Read the model definition and answer for the solid it produces. Units are mm, in the model's axes. A direction names the side the tool comes from. Coordinates: 2 decimals unless noted, no trailing zeros. Order: outer loops, then holes, each group sorted by start corner. A loop starts at its lowest first (then second) coordinate and runs counter-clockwise, first axis right, second up. Notation, with made-up numbers: (32, 70.5) -> (52, 70.5) arc R12 ccw to (52, 78.5) -> close; hole circle Ø5 at (-5, 69.25). An arc over 180 degrees is marked (long way). Use CSV: the item, a comma, the result in double quotes.
```python
from build123d import *

# Parameters (mm, degrees)
SKETCH_1_W           = 180
SKETCH_1_H           = 60
SKETCH_1_R           = 11
SKETCH_1_R_2         = 1.5
EXTRUDE_3_DEPTH      = 5
SKETCH_2_W           = 10
SKETCH_2_H           = 20
EXTRUDE_4_DEPTH      = 20
SKETCH_4_R           = 4
CUT_EXTRUDE_1_DEPTH  = 20
SKETCH_8_W           = 3
SKETCH_8_H           = 20
CUT_EXTRUDE_4_DEPTH  = 10
SKETCH_10_W          = 14
SKETCH_10_H          = 20
EXTRUDE_5_DEPTH      = 10
SKETCH_9_R           = 4
CUT_EXTRUDE_5_DEPTH  = 10
SKETCH_12_W          = 13.5
SKETCH_12_H          = 20
CUT_EXTRUDE_6_DEPTH  = 10
SKETCH_15_W          = 1
SKETCH_15_H          = 20
CUT_EXTRUDE_7_DEPTH  = 10
FILLET_5_R           = 5
SKETCH_21_W          = 10
SKETCH_21_H          = 18
EXTRUDE_6_DEPTH      = 20
SKETCH_23_R          = 4
CUT_EXTRUDE_9_DEPTH  = 20
FILLET_8_R           = 8
SKETCH_25_W          = 11.311173877
SKETCH_25_H          = 1.5
CUT_EXTRUDE_10_DEPTH = 20
FILLET_9_R           = 8
SKETCH_28_W          = 10
SKETCH_28_H          = 16.5
EXTRUDE_7_DEPTH      = 25
SKETCH_31_W          = 27.629977972
SKETCH_31_H          = 33.342762348
CUT_EXTRUDE_12_DEPTH = 20
SKETCH_33_W          = 10
SKETCH_33_H          = 20
EXTRUDE_8_DEPTH      = 6
SKETCH_34_W          = 10
SKETCH_34_H          = 20
CUT_EXTRUDE_13_DEPTH = 6
SKETCH_35_R          = 4
CUT_EXTRUDE_14_DEPTH = 10
FILLET_11_R          = 8
SKETCH_36_R          = 1.5
CUT_EXTRUDE_15_DEPTH = 10
SKETCH_37_R          = 4.5
CUT_EXTRUDE_16_DEPTH = 10
SKETCH_38_R          = 11.5
CUT_EXTRUDE_17_DEPTH = 10
SKETCH_39_R          = 1.5
CUT_EXTRUDE_18_DEPTH = 10
FILLET_13_R          = 8


with BuildPart() as part:
    # 스케치1 → 보스-돌출3 (new body)
    with BuildSketch(Plane(origin=(0, 0, 0), x_dir=(1, 0, 0), z_dir=(0, 1, 0))):
        with Locations((36.632340007, -1.742375967)):
            Rectangle(SKETCH_1_W, SKETCH_1_H)
        with Locations(Location((105.632340007, 7.257624033, 0), (0, 0, 270))):
            Circle(SKETCH_1_R, mode=Mode.SUBTRACT)
        with Locations(Location((90.132340007, 22.757624033, 0), (0, 0, 270))):
            Circle(SKETCH_1_R_2, mode=Mode.SUBTRACT)
        with Locations(Location((121.132340007, 22.757624033, 0), (0, 0, 270))):
            Circle(SKETCH_1_R_2, mode=Mode.SUBTRACT)
        with Locations(Location((90.132340007, -8.242375967, 0), (0, 0, 270))):
            Circle(SKETCH_1_R_2, mode=Mode.SUBTRACT)
        with Locations(Location((121.132340007, -8.242375967, 0), (0, 0, 270))):
            Circle(SKETCH_1_R_2, mode=Mode.SUBTRACT)
        with Locations(Location((-32.617755763, 4.712595626, 0), (0, 0, 270))):
            Circle(SKETCH_1_R_2, mode=Mode.SUBTRACT)
        with Locations(Location((-45.654401225, 19.548720133, 0), (0, 0, 270))):
            Circle(SKETCH_1_R_2, mode=Mode.SUBTRACT)
        with Locations(Location((-45.654401225, -10.123528882, 0), (0, 0, 270))):
            Circle(SKETCH_1_R_2, mode=Mode.SUBTRACT)
    extrude(amount=EXTRUDE_3_DEPTH)

    # 스케치2 → 보스-돌출4 (add)
    with BuildSketch(Plane(origin=(0, 5, 0), x_dir=(1, 0, 0), z_dir=(0, 1, 0))):
        with Locations((79.782459712, 8.257624033)):
            Rectangle(SKETCH_2_W, SKETCH_2_H)
    extrude(amount=EXTRUDE_4_DEPTH)

    # 스케치4 → 컷-돌출1 (cut)
    with BuildSketch(Plane.ZY.offset(-74.782459712)):
        with Locations((-8.257624033, 15)):
            Circle(SKETCH_4_R)
    extrude(amount=-CUT_EXTRUDE_1_DEPTH, mode=Mode.SUBTRACT)

    # 스케치8 → 컷-돌출4 (cut)
    with BuildSketch(Plane(origin=(84.782459712, 0, 0), x_dir=(0, 0, -1), z_dir=(1, 0, 0))):
        with Locations((16.757624033, 15)):
            Rectangle(SKETCH_8_W, SKETCH_8_H)
        with Locations((-0.242375967, 15)):
            Rectangle(SKETCH_8_W, SKETCH_8_H)
    extrude(amount=-CUT_EXTRUDE_4_DEPTH, mode=Mode.SUBTRACT)

    # 스케치10 → 보스-돌출5 (add)
    with BuildSketch(Plane(origin=(84.782459712, 0, 0), x_dir=(0, 0, -1), z_dir=(1, 0, 0))):
        with Locations((-5.242375967, 15)):
            Rectangle(SKETCH_10_W, SKETCH_10_H)
    extrude(amount=-EXTRUDE_5_DEPTH)

    # 스케치9 → 컷-돌출5 (cut)
    with BuildSketch(Plane(origin=(84.782459712, 0, 0), x_dir=(0, 0, -1), z_dir=(1, 0, 0))):
        with Locations((-5.242375967, 15)):
            Circle(SKETCH_9_R)
    extrude(amount=-CUT_EXTRUDE_5_DEPTH, mode=Mode.SUBTRACT)

    # 스케치12 → 컷-돌출6 (cut)
    with BuildSketch(Plane(origin=(84.782459712, 0, 0), x_dir=(0, 0, -1), z_dir=(1, 0, 0))):
        with Locations((8.507624033, 15)):
            Rectangle(SKETCH_12_W, SKETCH_12_H)
    extrude(amount=-CUT_EXTRUDE_6_DEPTH, mode=Mode.SUBTRACT)

    # 스케치15 → 컷-돌출7 (cut)
    with BuildSketch(Plane(origin=(84.782459712, 0, 0), x_dir=(0, 0, -1), z_dir=(1, 0, 0))):
        with Locations((1.257624033, 15)):
            Rectangle(SKETCH_15_W, SKETCH_15_H)
    extrude(amount=-CUT_EXTRUDE_7_DEPTH, mode=Mode.SUBTRACT)

    # 필렛5
    fillet_5_edges = [part.edges().sort_by_distance(p)[0] for p in [
        (79.782459712, 25, -0.757624033),
        (79.782459712, 25, 12.242375967),
    ]]
    fillet(fillet_5_edges, radius=FILLET_5_R)

    # 스케치21 → 보스-돌출6 (add)
    with BuildSketch(Plane(origin=(0, 5, 0), x_dir=(1, 0, 0), z_dir=(0, 1, 0))):
        with Locations((79.782459712, -5.742375967)):
            Rectangle(SKETCH_21_W, SKETCH_21_H)
    extrude(amount=EXTRUDE_6_DEPTH)

    # 스케치23 → 컷-돌출9 (cut)
    with BuildSketch(Plane(origin=(84.782459712, 0, 0), x_dir=(0, 0, -1), z_dir=(1, 0, 0))):
        with Locations((-5.742375967, 15)):
            Circle(SKETCH_23_R)
    extrude(amount=-CUT_EXTRUDE_9_DEPTH, mode=Mode.SUBTRACT)

    # 필렛8
    fillet_8_edges = [part.edges().sort_by_distance(p)[0] for p in [
        (79.782459712, 5, 14.742375967),
    ]]
    fillet(fillet_8_edges, radius=FILLET_8_R)

    # 스케치25 → 컷-돌출10 (cut)
    with BuildSketch(Plane(origin=(0, 5, 0), x_dir=(1, 0, 0), z_dir=(0, 1, 0))):
        with Locations((79.126872773, 2.507624033)):
            Rectangle(SKETCH_25_W, SKETCH_25_H)
    extrude(amount=CUT_EXTRUDE_10_DEPTH, mode=Mode.SUBTRACT)

    # 필렛9
    fillet_9_edges = [part.edges().sort_by_distance(p)[0] for p in [
        (79.782459712, 25, 14.742375967),
        (79.782459712, 25, -1.757624033),
    ]]
    fillet(fillet_9_edges, radius=FILLET_9_R)

    # 스케치28 → 보스-돌출7 (add)
    with BuildSketch(Plane(origin=(0, 5, 0), x_dir=(1, 0, 0), z_dir=(0, 1, 0))):
        with Locations((79.782459712, -6.492375967)):
            Rectangle(SKETCH_28_W, SKETCH_28_H)
    extrude(amount=-EXTRUDE_7_DEPTH)

    # 스케치31 → 컷-돌출12 (cut)
    with BuildSketch(Plane(origin=(0, 5, 0), x_dir=(1, 0, 0), z_dir=(0, 1, 0))):
        with Locations((71.963070495, -8.53095436)):
            Rectangle(SKETCH_31_W, SKETCH_31_H)
    extrude(amount=CUT_EXTRUDE_12_DEPTH, mode=Mode.SUBTRACT)

    # 스케치33 → 보스-돌출8 (add)
    with BuildSketch(Plane.XY.offset(14.742375967)):
        with Locations((79.782459712, -10)):
            Rectangle(SKETCH_33_W, SKETCH_33_H)
    extrude(amount=EXTRUDE_8_DEPTH)

    # 스케치34 → 컷-돌출13 (cut)
    with BuildSketch(Plane(origin=(0, 0, -1.757624033), x_dir=(-1, 0, 0), z_dir=(0, 0, -1))):
        with Locations((-79.782459712, -10)):
            Rectangle(SKETCH_34_W, SKETCH_34_H)
    extrude(amount=-CUT_EXTRUDE_13_DEPTH, mode=Mode.SUBTRACT)

    # 스케치35 → 컷-돌출14 (cut)
    with BuildSketch(Plane(origin=(84.782459712, 0, 0), x_dir=(0, 0, -1), z_dir=(1, 0, 0))):
        with Locations((-11.742375967, -10)):
            Circle(SKETCH_35_R)
    extrude(amount=-CUT_EXTRUDE_14_DEPTH, mode=Mode.SUBTRACT)

    # 필렛11
    fillet_11_edges = [part.edges().sort_by_distance(p)[0] for p in [
        (79.782459712, 0, 20.742375967),
        (79.782459712, -20, 20.742375967),
        (79.782459712, -20, 4.242375967),
    ]]
    fillet(fillet_11_edges, radius=FILLET_11_R)

    # 스케치36 → 컷-돌출15 (cut)
    with BuildSketch(Plane.XZ):
        with Locations(Location((-16.194092027, 6.822922113, 0), (0, 0, 270))):
            Circle(SKETCH_36_R)
        with Locations(Location((-16.114067961, -11.797077887, 0), (0, 0, 270))):
            Circle(SKETCH_36_R)
        with Locations(Location((0.805907973, 6.822922113, 0), (0, 0, 270))):
            Circle(SKETCH_36_R)
        with Locations(Location((0.885932039, -11.797077887, 0), (0, 0, 270))):
            Circle(SKETCH_36_R)
        with Locations(Location((17.805907973, 6.822922113, 0), (0, 0, 270))):
            Circle(SKETCH_36_R)
        with Locations(Location((17.885932039, -11.797077887, 0), (0, 0, 270))):
            Circle(SKETCH_36_R)
        with Locations(Location((34.805907973, 6.822922113, 0), (0, 0, 270))):
            Circle(SKETCH_36_R)
        with Locations(Location((34.885932039, -11.797077887, 0), (0, 0, 270))):
            Circle(SKETCH_36_R)
        with Locations(Location((51.805907973, 6.822922113, 0), (0, 0, 270))):
            Circle(SKETCH_36_R)
        with Locations(Location((51.885932039, -11.797077887, 0), (0, 0, 270))):
            Circle(SKETCH_36_R)
        with Locations(Location((68.805907973, 6.822922113, 0), (0, 0, 270))):
            Circle(SKETCH_36_R)
        with Locations(Location((68.885932039, -11.797077887, 0), (0, 0, 270))):
            Circle(SKETCH_36_R)
    extrude(amount=-CUT_EXTRUDE_15_DEPTH, mode=Mode.SUBTRACT)

    # 스케치37 → 컷-돌출16 (cut)
    with BuildSketch(Plane(origin=(84.782459712, 0, 0), x_dir=(0, 0, -1), z_dir=(1, 0, 0))):
        with Locations((-11.742375967, -10)):
            Circle(SKETCH_37_R)
    extrude(amount=-CUT_EXTRUDE_16_DEPTH, mode=Mode.SUBTRACT)

    # 스케치38 → 컷-돌출17 (cut)
    with BuildSketch(Plane.XZ):
        with Locations(Location((105.632340007, -7.257624033, 0), (0, 0, 270))):
            Circle(SKETCH_38_R)
    extrude(amount=-CUT_EXTRUDE_17_DEPTH, mode=Mode.SUBTRACT)

    # 스케치39 → 컷-돌출18 (cut)
    with BuildSketch(Plane(origin=(0, 0, 4.242375967), x_dir=(-1, 0, 0), z_dir=(0, 0, -1))):
        with Locations((-79.782459712, -9.106275905)):
            Circle(SKETCH_39_R)
    extrude(amount=-CUT_EXTRUDE_18_DEPTH, mode=Mode.SUBTRACT)

    # 필렛13
    fillet_13_edges = [part.edges().sort_by_distance(p)[0] for p in [
        (126.632340007, 2.5, -28.257624033),
        (126.632340007, 2.5, 31.742375967),
        (-53.367659993, 2.5, 31.742375967),
        (-53.367659993, 2.5, -28.257624033),
    ]]
    fillet(fillet_13_edges, radius=FILLET_13_R)


solid = part.part
```
Item 1: Find section B-B, the plane x = 12. Give the vertices of the cut face in (y, z).
Return value:
outline,"(0, -28.26) -> (5, -28.26) -> (5, 31.74) -> (0, 31.74) -> close"
Item 2: The mould has two halves that part along Z. Classify faces 4 (the flat face through (35, 2, 31.742)), 5 (the flat face through (84.782, -8, 16)), 6 (the cylindrical face through (33.34, 2.46, 7.15)): +Z half, -Z half, draft (parallel to the pull), parting line (faces both ways), or undercut.
Return value:
face 4,"+Z half"
face 5,"draft"
face 6,"undercut"
Item 3: Find section A-A, the plane z = 27. Give the vertices of the cut face in (x, y), then the cut area to 3 significant figures.
Return value:
outline,"(-52.67, 0) -> (74.78, 0) -> (74.78, -0.19) -> (84.78, -0.19) -> (84.78, 0) -> (125.94, 0) -> (125.94, 5) -> (-52.67, 5) -> close"
area,"895 mm^2"
Item 4: A tool of negligible diameter and unlimited length cuts with its end or side. For faces 1 (the flat face through (74.782, -8, 16)), 2 (the cylindrical face through (124.23, 2.54, 29.46)), 3 (the cylindrical face through (79.98, -7.62, 5.65)), from which of +Z, -Z, +X, -X, +Y, -Y can it reach the whole face along a straight path? Write none if from no direction.
Return value:
face 1,"+Z, -Z, -X, -Y"
face 2,"+Z, +X, +Y, -Y"
face 3,"-Z"
Item 5: Find section C-C, the plane y = -2.75. Give the vertices of the cut face in (x, z).
Return value:
outline,"(74.78, 4.24) -> (84.78, 4.24) -> (84.78, 22.71) -> (74.78, 22.71) -> close"
Item 6: Each of these flat-tipped pins is pushed along its axis until it touches: P1, Ø2, axis at x = 108.5, z = 18.5, coming from the -Y side; P2, Ø1.8, axis at x = 68.89, z = -11.8, coming from the -Y side (3 decimals); P3, Ø12, axis at x = 24.5, y = -5.5, coming from the +Z side; P4, Ø4.5, axis at x = 77.5, y = -9.5, coming from the +Z side. Where does it stop, or does it pass through?
Return value:
P1,"stops at y = 0"
P2,"passes through"
P3,"stops at z = 31.74"
P4,"stops at z = 20.78"
Item 7: Straight lines are drawn through the part: line 1 along Y through (x, z) = (46, -7.5); line 2 along X through (y, z) = (-15.5, 15.5); line 3 along X through (y, z) = (1.25, -19). For each, find the intervals that lie inside material, in ascending order.
Return value:
line 1,"y = 0 to 5"
line 2,"x = 74.78 to 84.78"
line 3,"x = -53.37 to -47.05, -44.26 to 126.63"
